Check sheet for the modelled part. Datum: model origin and axes. Units: mm. A direction names the side the tool comes from. Round coordinates to 2 decimals unless told otherwise and drop trailing zeros. Write each loop counter-clockwise with the first axis right and the second up, starting at its lowest first coordinate (ties: lowest second). Pieces come first, ordered by that corner, then holes. Notation, with made-up numbers: (62.25, -34.5) - (96.25, -34.5) arc R11 cw to (96.25, -18.5) - close; hole circle Ø11 at (19, -27.5). An arc over 180 degrees is marked (long way). Answer as a JSON object with one key per item and string values. Group by question number.
Item 1: Sectioned sample at D-D on x = 14. Record the boundary of the cut face in (y, z), plus the area to 3 significant figures.
Item 2: Sectioned sample at B-B on x = 5. Count the separate pieces of the cut face and the enclosed holes in it, plus the area to 3 significant figures.
Item 3: Set-up check for faces 1 (the flat face through (18, 9, 5)), 2 (the flat face through (18, 8, 0)): record each of +Z, -Z, +X, -X, +Y, -Y from which the full face is reachable in a straight line by a thin tool's end or side.
Item 4: Sectioned sample at C-C on z = -5. Record the boundary of the cut face in (x, y).
Item 5: Gauge pin test, flat ends, axial feed: P1, Ø5.5, axis at x = 31, y = 5, coming from the -Z side; P2, Ø3, axis at x = 31, z = -20, coming from the -Y side; P3, Ø4.5, axis at x = 31, y = 13, coming from the +Z side; P4, Ø12, axis at x = 25, z = -10, coming from the -Y side. Record the tip position at first contact, or that the pin passes through.
Item 6: Release check for a two-part mould opening along X. For faces 3 (the flat face through (18, 23, -14)), 4 (the flat face through (36, 18.3, -7.4)), 5 (the cylindrical face through (32.57, 21.25, -4.35)) record: pulls with the +X half, pulls with the -X half, needs draft (parallel to the pull), parting line crosses it, or undercut.
Item 7: Thickness scan on line 1 (X direction, y = 21.1, z = -20); line 2 (Z direction, x = 31, y = 21.95); line 3 (Y direction, x = 5, z = 3.8). Record the ranges inside material, lowest first.
Item 8: Sectioned sample at A-A on y = 13. Record the boundary of the cut face in (x, z), plus the area to 3 significant figures.
```python
from build123d import *

# Parameters (mm, degrees)
SKETCH1_W                                       = 36
SKETCH1_H                                       = 18
BOSS_EXTRUDE1_DEPTH                             = 5
CSK_FOR_M3_FLAT_HEAD_MACHINE_SCREW1_D           = 3.4
CSK_FOR_M3_FLAT_HEAD_MACHINE_SCREW1_DEPTH       = 5
CSK_FOR_M3_FLAT_HEAD_MACHINE_SCREW1_CSINK_D     = 6.3
CSK_FOR_M3_FLAT_HEAD_MACHINE_SCREW1_CSINK_ANGLE = 90
SKETCH7_W                                       = 36
SKETCH7_H                                       = 32
BOSS_EXTRUDE2_DEPTH                             = 5
CSK_FOR_M3_FLAT_HEAD_MACHINE_SCREW2_D           = 3.4
CSK_FOR_M3_FLAT_HEAD_MACHINE_SCREW2_DEPTH       = 5
CSK_FOR_M3_FLAT_HEAD_MACHINE_SCREW2_CSINK_D     = 6.3
CSK_FOR_M3_FLAT_HEAD_MACHINE_SCREW2_CSINK_ANGLE = 90
FILLET1_R                                       = 1.5
FILLET2_R                                       = 5


with BuildPart() as part:
    # Sketch1 → Boss-Extrude1 (new body)
    with BuildSketch(Plane.XY):
        with Locations((18, 9)):
            Rectangle(SKETCH1_W, SKETCH1_H)
    extrude(amount=BOSS_EXTRUDE1_DEPTH)

    # CSK for M3 Flat Head Machine Screw1
    with Locations(Plane(origin=(0, 0, 0), x_dir=(-1, 0, 0), z_dir=(0, 0, -1))):
        with Locations((-31, 13), (-31, 5), (-5, 5), (-5, 13)):
            CounterSinkHole(CSK_FOR_M3_FLAT_HEAD_MACHINE_SCREW1_D / 2, CSK_FOR_M3_FLAT_HEAD_MACHINE_SCREW1_CSINK_D / 2, depth=CSK_FOR_M3_FLAT_HEAD_MACHINE_SCREW1_DEPTH, counter_sink_angle=CSK_FOR_M3_FLAT_HEAD_MACHINE_SCREW1_CSINK_ANGLE)

    # Sketch7 → Boss-Extrude2 (add)
    with BuildSketch(Plane(origin=(0, 18, 0), x_dir=(1, 0, 0), z_dir=(0, 1, 0))):
        with Locations((18, 11)):
            Rectangle(SKETCH7_W, SKETCH7_H)
    extrude(amount=BOSS_EXTRUDE2_DEPTH)

    # CSK for M3 Flat Head Machine Screw2
    with Locations(Plane(origin=(0, 18, 0), x_dir=(-1, 0, 0), z_dir=(0, -1, 0))):
        with Locations((-31, 5), (-31, 20), (-5, 20), (-5, 5)):
            CounterSinkHole(CSK_FOR_M3_FLAT_HEAD_MACHINE_SCREW2_D / 2, CSK_FOR_M3_FLAT_HEAD_MACHINE_SCREW2_CSINK_D / 2, depth=CSK_FOR_M3_FLAT_HEAD_MACHINE_SCREW2_DEPTH, counter_sink_angle=CSK_FOR_M3_FLAT_HEAD_MACHINE_SCREW2_CSINK_ANGLE)

    # Fillet1
    fillet1_edges = [part.edges().sort_by_distance(p)[0] for p in [
        (18, 18, 0),
    ]]
    fillet(fillet1_edges, radius=FILLET1_R)

    # Fillet2
    fillet2_edges = [part.edges().sort_by_distance(p)[0] for p in [
        (18, 23, 5),
    ]]
    fillet(fillet2_edges, radius=FILLET2_R)


solid = part.part
```
Completed:
{
 "1": {"outline": "(0, 0) - (16.5, 0) arc R1.5 cw to (18, -1.5) - (18, -27) - (23, -27) - (23, 0) arc R5 ccw to (18, 5) - (0, 5) - close", "area": "245 mm²"},
 "2": {"separate pieces": "5", "enclosed holes": "0", "area": "169 mm²"},
 "3": {"face 1": "+Z, +X, -X, +Y, -Y", "face 2": "-Z, +X, -X, -Y"},
 "4": {"outline": "(0, 18) - (1.85, 18) - (3.3, 19.45) - (3.3, 23) - (0, 23) - close; (6.7, 19.45) - (8.15, 18) - (27.85, 18) - (29.3, 19.45) - (29.3, 23) - (6.7, 23) - close; (32.7, 19.45) - (34.15, 18) - (36, 18) - (36, 23) - (32.7, 23) - close"},
 "5": {"P1": "z = 0.4", "P2": "through", "P3": "z = 5", "P4": "y = 18"},
 "6": {"face 3": "needs draft", "face 4": "pulls with the +X half", "face 5": "undercut"},
 "7": {"line 1": "0 to 3.3, 6.7 to 29.3, 32.7 to 36", "line 2": "-27 to -21.7, -18.3 to -6.7, -3.3 to 3.07", "line 3": "0 to 3.3, 6.7 to 11.3, 14.7 to 21.25"},
 "8": {"outline": "(0, 0) - (1.85, 0) - (3.3, 1.45) - (3.3, 5) - (0, 5) - close; (6.7, 1.45) - (8.15, 0) - (27.85, 0) - (29.3, 1.45) - (29.3, 5) - (6.7, 5) - close; (32.7, 1.45) - (34.15, 0) - (36, 0) - (36, 5) - (32.7, 5) - close", "area": "142 mm²"}
}
